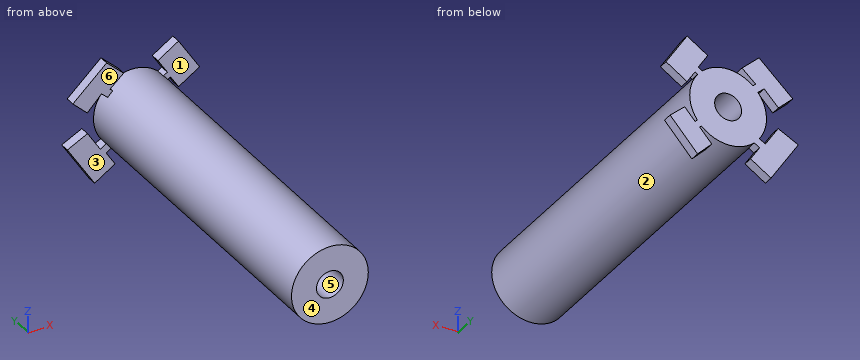
from build123d import *

# Parameters (mm, degrees)
F0_R     = 4
F0_R_2   = 1.4
F1_DEPTH = 35
F4_DEPTH = 1


with BuildPart() as f1:
    # F0 (on Front) → F1 (new body)
    with BuildSketch(Plane.XZ):
        Circle(F0_R)
        Circle(F0_R_2, mode=Mode.SUBTRACT)
    extrude(amount=F1_DEPTH)

    # F3 (on face) → F4 (join)
    with BuildSketch(Plane(origin=(0, 0, 0), x_dir=(-1, 0, 0), z_dir=(0, 1, 0))):
        Polygon((-3.441267, 2.621837), (-2.658013, 2.116282), (-2.527552, 2.052343), (-2.159969, 2.621837), (-3.109507, 3.23472), (-2.119805, 4.768063), (-4.266258, 6.153501), (-6.466136, 2.745238), (-4.274626, 1.330718), align=None)
        Polygon((-2.259792, -2.418553), (-2.658013, -1.912313), (-3.441267, -2.611758), (-4.519502, -1.404327), (-6.038423, -2.760721), (-3.180103, -5.961532), (-1.700384, -4.458029), (-2.961811, -3.045455), align=None)
        Polygon((3.877339, -2.704357), (2.650228, -1.912313), (2.136546, -2.549902), (3.276904, -3.285951), (2.340704, -4.736403), (4.467671, -6.109263), (7.312901, -1.701158), (5.213581, -0.634123), align=None)
        Polygon((2.864772, 3.32476), (2.136546, 2.621837), (2.650228, 2.116282), (3.755631, 3.103405), (5.239515, 1.551226), (6.736414, 2.982262), (3.221487, 6.206864), (1.448484, 4.569151), align=None)
    extrude(amount=-F4_DEPTH)


solid = f1.part
Verification items for the finished model (mm, model axes). Face numbers are marked on the shaded views. A direction names the side the tool comes from. Round coordinates to 2 decimals unless told otherwise and drop trailing zeros. Loops run counter-clockwise (first coordinate to the right, second up) from the corner with the lowest first, then second, coordinate; pieces in that order, holes last. Notation, with made-up numbers: (-13, 45.5) - (20, 45.5) arc R9 cw to (20, 59.5) - close; hole circle Ø6 at (16, 52.25). An arc over 180 degrees is marked (long way). Use a Markdown table: item, result. Add a question column.
1. Section check C-C, the plane y = -10. Record the boundary of the cut face in (x, z).
2. Section check A-A, the plane z = 0. Record the boundary of the cut face in (x, y), plus the area to 3 significant figures.
3. Gauge pin test, flat ends, axial feed: pin 1 (4 mm diameter, centred on y = -17.5, z = 0.5, fed in from +X); pin 2 (1.5 mm diameter, centred on x = -4, y = -25.5, fed in from +Z); pin 3 (5 mm diameter, centred on x = -2, y = -16, fed in from +Z); pin 4 (1.7 mm diameter, centred on x = 0, z = 0, fed in from -Y). Record the tip position at first contact, or that the pin passes through.
4. Thickness scan on probe 1 along Z at (x, y) = (0, -10); probe 2 along Z at (x, y) = (-1, -14.5); probe 3 along X at (y, z) = (-26, 0.25). Record the ranges inside material, lowest first. Write a range as [from, to].
5. Access from +Z, -Z, +X, -X, +Y, -Y to the whole of each face (thin tool, end or side, straight path). Record for the marked faces 1, 2, 3 and 4.
6. Release check for a two-part mould opening along Z. For the marked faces 5 and 6 record: released by +Z, released by -Z, zero draft, split by the parting line, or undercut.
7. Section check B-B, the plane x = 0. Record the boundary of the cut face in (y, z).
Checks:
| question | item | result |
|---|---|---|
| 1 | outline | circle Ø8 at (0, 0); hole circle Ø2.8 at (0, 0) |
| 2 | outline | (-4, -35) - (-1.4, -35) - (-1.4, 0) - (-4, 0) - close; (1.4, -35) - (4, -35) - (4, 0) - (1.4, 0) - close |
| 2 | area | 182 mm^2 |
| 3 | pin 1 | stops at x = 4 |
| 3 | pin 2 | stops at z = 2.33 |
| 3 | pin 3 | stops at z = 4 |
| 3 | pin 4 | passes through |
| 4 | probe 1 | z = [-4, -1.4], [1.4, 4] |
| 4 | probe 2 | z = [-3.87, -0.98], [0.98, 3.87] |
| 4 | probe 3 | x = [-3.99, -1.38], [1.38, 3.99] |
| 5 | face 1 | +Z, +X, -Y |
| 5 | face 2 | -Y |
| 5 | face 3 | -Z, -X, -Y |
| 5 | face 4 | +Z, -Z, +X, -X, -Y |
| 6 | face 5 | undercut |
| 6 | face 6 | zero draft |
| 7 | outline | (-35, -4) - (0, -4) - (0, -1.4) - (-35, -1.4) - close; (-35, 1.4) - (0, 1.4) - (0, 4) - (-35, 4) - close |
